from build123d import *

# Parameters (mm, degrees)
F1_ANGLE = 180
F3_DEPTH = 127
F6_R     = 2
F7_R     = 2


with BuildPart() as f1:
    # F0 (on Front) → F1 (revolve)
    with BuildSketch(Plane.XZ):
        with BuildLine():
            Line((5.25, 63.5), (-5.25, 63.5))
            Line((-5.25, 63.5), (-5.25, 20))
            add(Edge.make_bspline(
                [(-5.25, 20), (-5.8853452496, 14.3080799964), (-7.0077819126, 4.2524138852), (-7.0249760105, -5.1144951824), (-5.8863231474, -14.6635947641), (-5.25, -20)],
                knots=[0, 0, 0, 0, 0.3652549784, 0.6452799944, 1, 1, 1, 1], degree=3))
            Line((-5.25, -20), (-5.25, -63.5))
            Line((-5.25, -63.5), (5.25, -63.5))
            Line((5.25, -63.5), (5.25, 63.5))
        make_face()
    revolve(axis=Axis((5.25, 0, 0), (0, 0, -1)), revolution_arc=F1_ANGLE)

    # F2 (on face) → F3 (cut)
    with BuildSketch(Plane.XY.offset(63.5)):
        with BuildLine():
            Line((-1.75, 0), (5.25, 0))
            Line((5.25, 0), (12.25, 0))
            Line((12.25, 0), (12.25, 0.7))
            ThreePointArc((12.25, 0.7), (12.1621320344, 0.9121320344), (11.95, 1))
            Line((11.95, 1), (-1.45, 1))
            ThreePointArc((-1.45, 1), (-1.6621320344, 0.9121320344), (-1.75, 0.7))
            Line((-1.75, 0.7), (-1.75, 0))
        make_face()
    extrude(amount=-F3_DEPTH, mode=Mode.SUBTRACT)


with BuildPart() as f4_1:
    # F4: instance of F1
    add(f1.part.mirror(Plane.XZ))

    # F6
    f6_edges = [f4_1.edges().sort_by_distance(p)[0] for p in [
        (5.25, -10.5, 63.5),
    ]]
    fillet(f6_edges, radius=F6_R)

    # F7
    f7_edges = [f4_1.edges().sort_by_distance(p)[0] for p in [
        (5.25, -10.5, -63.5),
    ]]
    fillet(f7_edges, radius=F7_R)


solid = f4_1.part
Geometry: final body of the model. Coordinates: model frame, mm. A direction names the side the tool comes from. Coordinates: 2 decimals unless noted, no trailing zeros. Loops run counter-clockwise (first coordinate to the right, second up) from the corner with the lowest first, then second, coordinate; pieces in that order, holes last. Notation, with made-up numbers: M 54,-19 L 67,-19 A23 ccw 67,10 Z; hole C 43,-35.5 d5. An arc over 180 degrees is marked long. One line per item, written item: value. Start each with the question number.
1) Pin query (flat end, axial travel): P1, Ø2, axis at y = -2.5, z = 20, coming from the +X side; P2, Ø10.5, axis at x = 6.5, z = 10, coming from the +Y side; P3, Ø0.6, axis at y = -0.5, z = 10.5, coming from the +X side. Return the tip coordinate at first contact, or that it passes through.
2) Reachability of faces 1 (the cylindrical face through (5.019, -10.497, 40.46)), 2 (the flat face through (5, -4, -63.5)), 3 (the cylindrical face through (5.019, -10.497, -41.04)), 4 (the flat face through (5, -1, 1)), 5 (the flat face through (14, 0, 1)) from +Z, -Z, +X, -X, +Y, -Y: full face, straight path, thin tool, end or side. Return the list, or none.
3) Cut plane A-A (z = 28). Return loops of the section in (x, y), then the cut area to 3 significant figures.
4) Material intervals for L1, parallel to Y at x = 5.5, z = -21; L2, parallel to Y at x = -2, z = 5.5; L3, parallel to X at y = -8.5, z = -9.5, sorted ascending. Write a range as from..to.
Evaluation:
1. P1: x = 15.68
1. P2: y = -1
1. P3: x = 16.79
2. face 1: +Z, -Y
2. face 2: -Z, +X, -X, +Y, -Y
2. face 3: -Z, -Y
2. face 4: +Z, -Z, +Y
2. face 5: +Z, -Z, +X, -X, +Y
3. outline: M -5.25,0 A10.5 ccw 15.75,0 L 12.25,0 L 12.25,-0.7 A0.3 cw 11.95,-1 L -1.45,-1 A0.3 cw -1.75,-0.7 L -1.75,0 Z
3. area: 159 mm^2
4. L1: -10.5..-1
4. L2: -9.51..0
4. L3: -2.76..13.26
